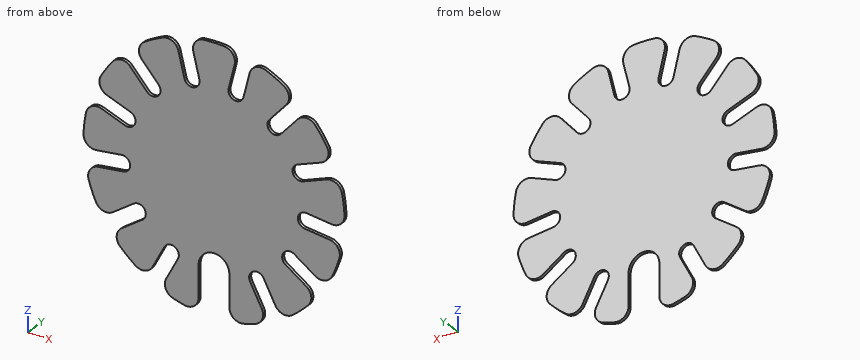
```python
from build123d import *

# Parameters (mm, degrees)
BOSS_EXTRUDE1_DEPTH     = 0.1
CUT_EXTRUDE1_DEPTH      = 1.1
CUT_EXTRUDE1_DEPTH_BACK = 1.1
FILLET1_R               = 0.75


with BuildPart() as part:
    # Sketch1 → Boss-Extrude1 (new body, symmetric)
    with BuildSketch(Plane(origin=(0, 0, 0), x_dir=(1, 0, 0), z_dir=(0, 1, 0))):
        with BuildLine():
            Line((-0.5, 6), (-0.5, 8.485281374))
            ThreePointArc((-0.5, 8.485281374), (-2.034183146, 8.253005448), (-3.500578863, 7.745705108))
            Line((-3.500578863, 7.745705108), (-2.345611019, 5.54509774))
            ThreePointArc((-2.345611019, 5.54509774), (-2.555977446, 4.870008141), (-3.231067045, 5.080374568))
            Line((-3.231067045, 5.080374568), (-4.386034889, 7.280981936))
            ThreePointArc((-4.386034889, 7.280981936), (-5.636542595, 6.362341359), (-6.699217295, 5.231681148))
            Line((-6.699217295, 5.231681148), (-4.653870822, 3.819880413))
            ThreePointArc((-4.653870822, 3.819880413), (-4.526411262, 3.124356107), (-5.221935569, 2.996896547))
            Line((-5.221935569, 2.996896547), (-7.267282042, 4.408697282))
            ThreePointArc((-7.267282042, 4.408697282), (-7.947638063, 3.01414154), (-8.363145779, 1.519142085))
            Line((-8.363145779, 1.519142085), (-5.895984904, 1.219574519))
            ThreePointArc((-5.895984904, 1.219574519), (-5.459898808, 0.662951741), (-6.016521585, 0.226865644))
            Line((-6.016521585, 0.226865644), (-8.48368246, 0.526433211))
            ThreePointArc((-8.48368246, 0.526433211), (-8.43802543, -1.024561782), (-8.111178352, -2.541414122))
            Line((-8.111178352, -2.541414122), (-5.7873999, -1.660121201))
            ThreePointArc((-5.7873999, -1.660121201), (-5.142589335, -1.950326879), (-5.432795013, -2.595137444))
            Line((-5.432795013, -2.595137444), (-7.756573465, -3.476430365))
            ThreePointArc((-7.756573465, -3.476430365), (-6.99536286, -4.828550347), (-6.001037715, -6.019762981))
            Line((-6.001037715, -6.019762981), (-4.352991324, -4.15950316))
            ThreePointArc((-4.352991324, -4.15950316), (-3.64717462, -4.116809115), (-3.604480575, -4.822625818))
            Line((-3.604480575, -4.822625818), (-5.252526967, -6.682885639))
            ThreePointArc((-5.252526967, -6.682885639), (-3.950146962, -7.526376218), (-2.516131657, -8.119056687))
            Line((-2.516131657, -8.119056687), (-1.921364894, -5.705993072))
            ThreePointArc((-1.921364894, -5.705993072), (-1.316236154, -5.340179996), (-0.950423077, -5.945308737))
            Line((-0.950423077, -5.945308737), (-1.54518984, -8.358372351))
            ThreePointArc((-1.54518984, -8.358372351), (0, -8.5), (1.54518984, -8.358372351))
            Line((1.54518984, -8.358372351), (0.950423077, -5.945308737))
            ThreePointArc((0.950423077, -5.945308737), (1.316236154, -5.340179996), (1.921364894, -5.705993072))
            Line((1.921364894, -5.705993072), (2.516131657, -8.119056687))
            ThreePointArc((2.516131657, -8.119056687), (3.950146962, -7.526376218), (5.252526967, -6.682885639))
            Line((5.252526967, -6.682885639), (3.604480575, -4.822625818))
            ThreePointArc((3.604480575, -4.822625818), (3.64717462, -4.116809115), (4.352991324, -4.15950316))
            Line((4.352991324, -4.15950316), (6.001037715, -6.019762981))
            ThreePointArc((6.001037715, -6.019762981), (6.99536286, -4.828550347), (7.756573465, -3.476430365))
            Line((7.756573465, -3.476430365), (5.432795013, -2.595137444))
            ThreePointArc((5.432795013, -2.595137444), (5.142589335, -1.950326879), (5.7873999, -1.660121201))
            Line((5.7873999, -1.660121201), (8.111178352, -2.541414122))
            ThreePointArc((8.111178352, -2.541414122), (8.43802543, -1.024561782), (8.48368246, 0.526433211))
            Line((8.48368246, 0.526433211), (6.016521585, 0.226865644))
            ThreePointArc((6.016521585, 0.226865644), (5.459898808, 0.662951741), (5.895984904, 1.219574519))
            Line((5.895984904, 1.219574519), (8.363145779, 1.519142085))
            ThreePointArc((8.363145779, 1.519142085), (7.947638063, 3.01414154), (7.267282042, 4.408697282))
            Line((7.267282042, 4.408697282), (5.221935569, 2.996896547))
            ThreePointArc((5.221935569, 2.996896547), (4.526411262, 3.124356107), (4.653870822, 3.819880413))
            Line((4.653870822, 3.819880413), (6.699217295, 5.231681148))
            ThreePointArc((6.699217295, 5.231681148), (5.636542595, 6.362341359), (4.386034889, 7.280981936))
            Line((4.386034889, 7.280981936), (3.231067045, 5.080374568))
            ThreePointArc((3.231067045, 5.080374568), (2.555977446, 4.870008141), (2.345611019, 5.54509774))
            Line((2.345611019, 5.54509774), (3.500578863, 7.745705108))
            ThreePointArc((3.500578863, 7.745705108), (2.034183146, 8.253005448), (0.5, 8.485281374))
            Line((0.5, 8.485281374), (0.5, 6))
            ThreePointArc((0.5, 6), (0, 5.5), (-0.5, 6))
        make_face()
    extrude(amount=BOSS_EXTRUDE1_DEPTH, both=True)

    # Sketch2 → Cut-Extrude1 (cut, two sides)
    with BuildSketch(Plane(origin=(0, 0, 0), x_dir=(1, 0, 0), z_dir=(0, 1, 0))) as cut_extrude1_sk:
        with BuildLine():
            Line((-1, 5.5), (-1, 8.485281374))
            Line((-1, 8.485281374), (1, 8.485281374))
            Line((1, 8.485281374), (1, 5.5))
            ThreePointArc((1, 5.5), (0, 4.5), (-1, 5.5))
        make_face()
    extrude(amount=CUT_EXTRUDE1_DEPTH, mode=Mode.SUBTRACT)
    extrude(cut_extrude1_sk.sketch, amount=-CUT_EXTRUDE1_DEPTH_BACK, mode=Mode.SUBTRACT)

    # Fillet1
    fillet1_edges = [part.edges().sort_by_distance(p)[0] for p in [
        (-1, 0, -8.440971508),
        (1, 0, -8.440971508),
        (3.500578863, 0, -7.745705108),
        (4.386034889, 0, -7.280981936),
        (6.699217295, 0, -5.231681148),
        (7.267282042, 0, -4.408697282),
        (8.363145779, 0, -1.519142085),
        (8.48368246, 0, -0.526433211),
        (8.111178352, 0, 2.541414122),
        (7.756573465, 0, 3.476430365),
        (6.001037715, 0, 6.019762981),
        (5.252526967, 0, 6.682885639),
        (2.516131657, 0, 8.119056687),
        (1.54518984, 0, 8.358372351),
        (-1.54518984, 0, 8.358372351),
        (-2.516131657, 0, 8.119056687),
        (-5.252526967, 0, 6.682885639),
        (-6.001037715, 0, 6.019762981),
        (-7.756573465, 0, 3.476430365),
        (-8.111178352, 0, 2.541414122),
        (-8.48368246, 0, -0.526433211),
        (-8.363145779, 0, -1.519142085),
        (-7.267282042, 0, -4.408697282),
        (-6.699217295, 0, -5.231681148),
        (-4.386034889, 0, -7.280981936),
        (-3.500578863, 0, -7.745705108),
    ]]
    fillet(fillet1_edges, radius=FILLET1_R)


solid = part.part
```
Here's how the part is built. I have some questions about the finished solid (model axes, mm). Coordinates: 2 decimals unless noted, no trailing zeros. Order: outer loops, then holes, each group sorted by start corner. A loop starts at its lowest first (then second) coordinate and runs counter-clockwise, first axis right, second up.
1) I need wall thicknesses on line 1 (X direction, y = 0, z = 3.5); line 2 (Z direction, x = -4.75, y = -0.05) (3 decimals); line 3 (Z direction, x = -7.5, y = 0.05). Which ranges of each line are inside material? Lowest first, please.
2) Imagine slicing it at B-B on z = 3.75. List the corners of the cut face in (x, y) for me, and give its area (3 significant figures).
3) Imagine slicing it at A-A on x = 0. List the corners of the cut face in (y, z) for me.
Response values:
1. line 1: x = -7.35 to 7.35
1. line 2: z = -6.936 to -3.886, -2.945 to 4.608, 6.123 to 6.985
1. line 3: z = -3.88 to -1.41, -0.41 to 2.29
2. outline: (-7.45, -0.1) - (7.45, -0.1) - (7.45, 0.1) - (-7.45, 0.1) - close
2. area: 2.98 mm2
3. outline: (-0.1, -4.5) - (0.1, -4.5) - (0.1, 8.5) - (-0.1, 8.5) - close
